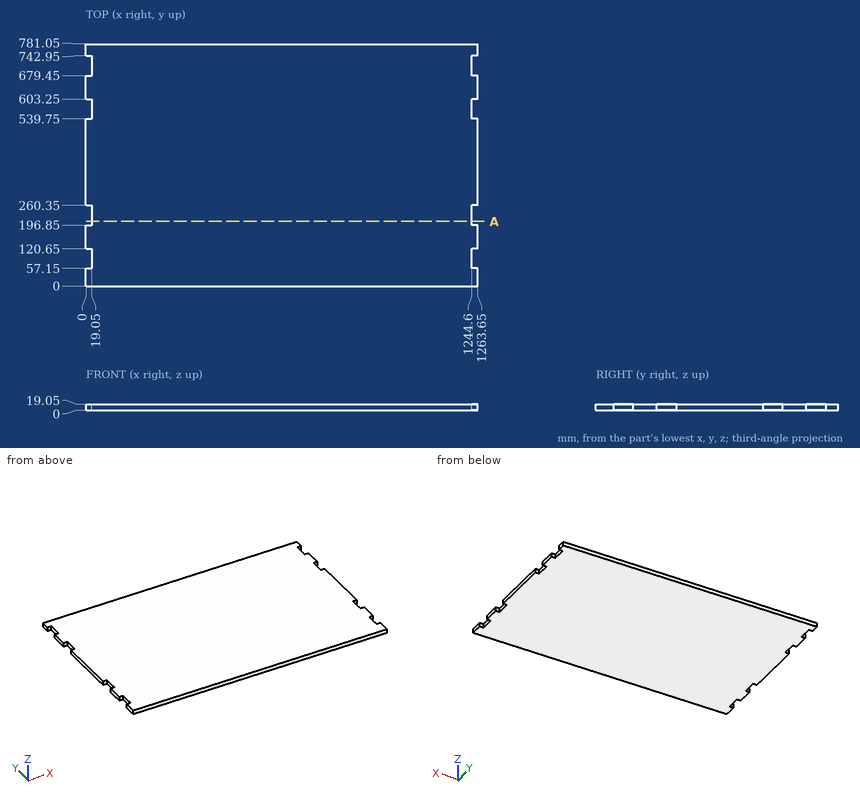
Geometry check sheet. Reference: drawing and pictorial views, mm from the part's lowest x, y, z. Round coordinates to 2 decimals unless told otherwise and drop trailing zeros. Loops run counter-clockwise (first coordinate to the right, second up) from the corner with the lowest first, then second, coordinate; pieces in that order, holes last. Notation, with made-up numbers: M 31,-16.75 L 37,-16.75 A11 ccw 37,-5.75 Z; hole C 11.5,33.25 d1. An arc over 180 degrees is marked long. Return JSON: item names as keys, results as strings. Group by question number.
(1) Scan line: line 1 along X through (y, z) = (221, 2). Record every from-to range of solid material in increasing order. Write a range as [from, to].
(2) Section check A-A, the plane y = 209. Enter the section's corners in (x, z), and give its area (3 significant figures).
(3) Go/stop test with flat-tipped pins: pin 1 (5.5 mm diameter, centred on y = 567, z = 12, fed in from +X); pin 2 (5.5 mm diameter, centred on y = 101.5, z = 10, fed in from -X). Record where each tip stops, or that it passes through.
Data:
{
 "1": {"line 1": "[19.05, 1244.6]"},
 "2": {"outline": "M 19.05,0 L 1244.6,0 L 1244.6,19.05 L 19.05,19.05 Z", "area": "23,300 mm²"},
 "3": {"pin 1": "x = 1244.6", "pin 2": "x = 19.05"}
}
